from build123d import *

# Parameters (mm, degrees)
CIRPATTERN1_COUNT = 2
CIRPATTERN1_ANGLE = 90


with BuildPart() as part:
    # BodySke → Base-Revolve (revolve)
    with BuildSketch(Plane.XY, mode=Mode.PRIVATE) as base_revolve_sk:
        with BuildLine():
            Line((4.6482, 3.96875), (4.6482, 8.8646))
            Line((4.6482, 8.8646), (4.113809896, 8.8646))
            ThreePointArc((4.113809896, 8.8646), (1.078560731, 4.886321853), (0, 0))
            Line((0, 0), (23.6982, 0))
            Line((23.6982, 0), (23.6982, 3.96875))
            Line((23.6982, 3.96875), (4.6482, 3.96875))
        make_face()
    revolve(base_revolve_sk.sketch.rotate(Axis((-25.4, 0, 0), (1, 0, 0)), 90), axis=Axis((-25.4, 0, 0), (1, 0, 0)))

    # Sketch3 → Cross section 0
    with BuildSketch(Plane(origin=(0, 0, 0), x_dir=(0, 0, -1), z_dir=(1, 0, 0))):
        with BuildLine():
            Line((0.8509, -4.9657), (-0.8509, -4.9657))
            Line((-0.8509, -4.9657), (-0.8509, 4.9657))
            Line((-0.8509, 4.9657), (0.8509, 4.9657))
            Line((0.8509, 4.9657), (0.8509, -4.9657))
        make_face()
    # Sketch4 → Cross section 1
    with BuildSketch(Plane(origin=(5.7912, 0, 0), x_dir=(0, 0, -1), z_dir=(1, 0, 0))):
        with BuildLine():
            Line((0.42545, -0.42545), (-0.42545, -0.42545))
            Line((-0.42545, -0.42545), (-0.42545, 0.42545))
            Line((-0.42545, 0.42545), (0.42545, 0.42545))
            Line((0.42545, 0.42545), (0.42545, -0.42545))
        make_face()
    cross = loft(mode=Mode.SUBTRACT)

    # CirPattern1: Cross ×2 about axis
    cirpattern1_axis = Axis((0, 0, 0), (1, 0, 0))
    for i in range(1, CIRPATTERN1_COUNT):
        add(cross.rotate(cirpattern1_axis, i * CIRPATTERN1_ANGLE / (CIRPATTERN1_COUNT - 1)), mode=Mode.SUBTRACT)


solid = part.part
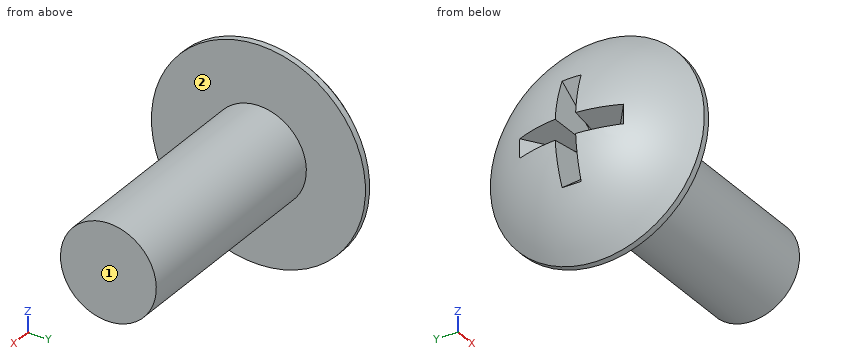
Verification items for the finished model (mm, model axes). Face numbers are marked on the shaded views. A direction names the side the tool comes from. Give positions to 0.01 mm unless a question says otherwise; leave off trailing zeros. Order: outer loops, then holes, each group sorted by start corner. A loop starts at its lowest first (then second) coordinate and runs counter-clockwise, first axis right, second up. Notation, with made-up numbers: M 19,78.5 L 60,78.5 A18 ccw 60,100.5 Z; hole C -15.75,-18.75 d6. An arc over 180 degrees is marked long. Answer as a JSON object with one key per item and string values. Group by question number.
1) Access from +Z, -Z, +X, -X, +Y, -Y to the whole of each face (thin tool, end or side, straight path). Record for the marked faces 1 and 2.
2) Cross-section at A-A (x = 8.25). Enter the section's corners in (y, z).
3) Cross-section at C-C (y = 5.25). Enter the section's corners in (x, z).
4) Scan lines: line 1 along X through (y, z) = (-4.5, -7.5); line 2 along Y through (x, z) = (2, -2.5); line 3 along Z through (x, y) = (8.5, -2.5). Record each from-to range of solid material in increasing order. Write a range as [from, to].
5) Cross-section at B-B (z = 6). Enter the section's corners in (x, y).
6) Depth check by flat-ended pin: pin 1 Ø5 at (y, z) = (-3.5, 6) entering from -X; pin 2 Ø10 at (x, y) = (17, 3.5) entering from -Z; pin 3 Ø5 at (x, y) = (20.5, -3.5) entering from +Z; pin 4 Ø8 at (x, z) = (5, -3.5) entering from -Y. Enter the tip coordinate at first touch or a pass-through.
Result sheet:
{
 "1": {"face 1": "+Z, -Z, +X, +Y, -Y", "face 2": "+X"},
 "2": {"outline": "C 0,0 d7.94"},
 "3": {"outline": "M 4.11,-7.14 L 4.65,-7.14 L 4.65,7.14 L 4.11,7.14 A10.35 ccw Z"},
 "4": {"line 1": "x = [3.98, 4.65]", "line 2": "y = [-6.02, -0.7], [0.7, 6.02]", "line 3": "z = [-3.08, 3.08]"},
 "5": {"outline": "M 4.11,-6.53 L 4.65,-6.53 L 4.65,6.53 L 4.11,6.53 A9.94 ccw Z"},
 "6": {"pin 1": "stops at x = 0.89", "pin 2": "stops at z = -3.97", "pin 3": "stops at z = 3.84", "pin 4": "stops at y = -8.86"}
}
